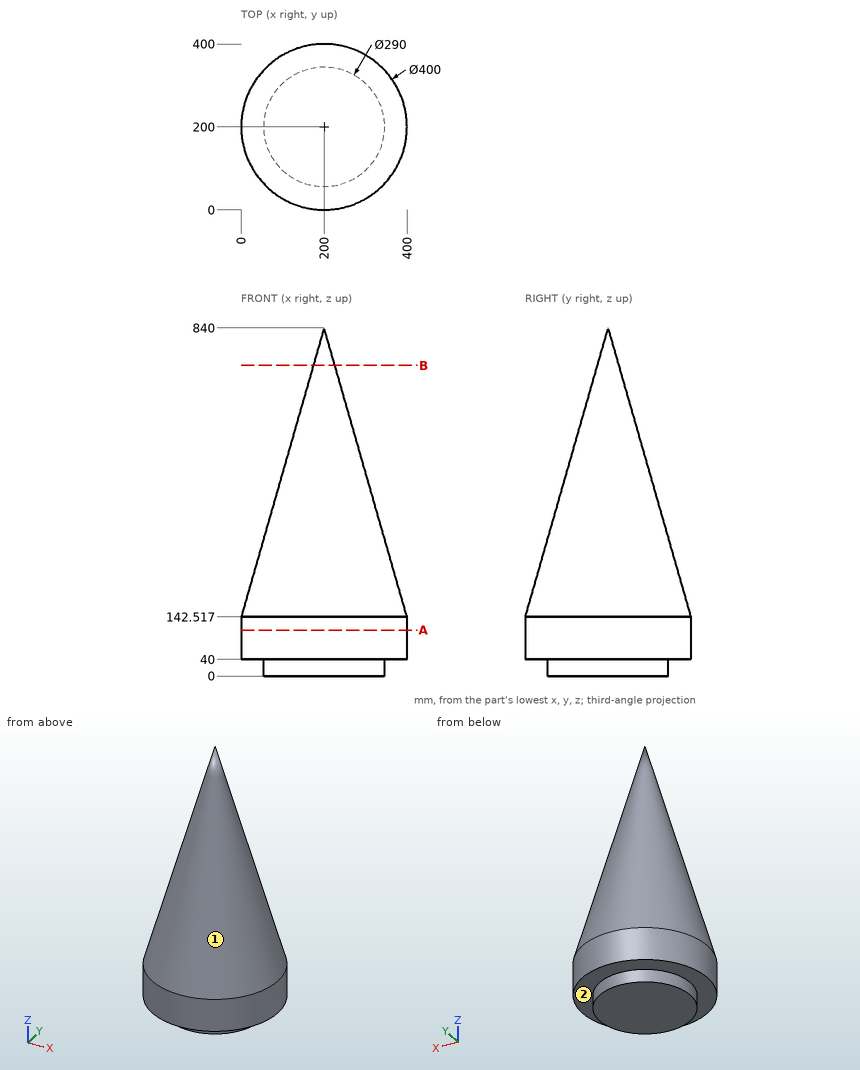
Part print with two shaded views. Sizes in mm from the minimum x, y, z corner. A direction names the side the tool comes from. Round coordinates to 2 decimals unless told otherwise and drop trailing zeros. Order: outer loops, then holes, each group sorted by start corner. A loop starts at its lowest first (then second) coordinate and runs counter-clockwise, first axis right, second up. Notation, with made-up numbers: M 74.5,10 L 94.5,10 A26 cw 94.5,24 Z; hole C 78,20 d8. An arc over 180 degrees is marked long. Answer in a Markdown table with one row per item. Add a question column.
Q1. Pin check, flat tips, straight feed: pin 1 (2 mm diameter, centred on y = 248, z = 204, fed in from -X); pin 2 (2 mm diameter, centred on x = 118.5, z = 157.5, fed in from -Y); pin 3 (10 mm diameter, centred on y = 152, z = 374, fed in from +X). Stop position of each tip, or through.
Q2. Cut at B-B on z = 749.5. Give the cut face in (x, y).
Q3. Cut at A-A on z = 110.5. Give the cut face in (x, y).
Q4. Wall check: L1, parallel to X at y = 199, z = 109.5; L2, parallel to Z at x = 62.5, y = 61.5; L3, parallel to Y at x = 66, z = 163.5. Give the ranges that are in metal, low to high. Write a range as from..to.
Q5. 3-axis set-ups, long thin cutter, end or side, ignore diameter. For the marked faces 1 and 2: which of +Z, -Z, +X, -X, +Y, -Y reach the whole face in a straight line?
Established:
| question | item | result |
|---|---|---|
| 1 | pin 1 | stops at x = 23.66 |
| 1 | pin 2 | stops at y = 21.52 |
| 1 | pin 3 | stops at x = 327.09 |
| 2 | outline | C 200,200 d51.9 |
| 3 | outline | C 200,200 d400 |
| 4 | L1 | x = 0..400 |
| 4 | L2 | z = 40..159.39 |
| 4 | L3 | y = 59.74..340.26 |
| 5 | face 1 | +Z |
| 5 | face 2 | -Z |
